Source: CAD feature listing. Evaluate the final solid. Frame: model axes, mm. A direction names the side the tool comes from. Give positions to 0.01 mm unless a question says otherwise; leave off trailing zeros. Order: outer loops, then holes, each group sorted by start corner. A loop starts at its lowest first (then second) coordinate and runs counter-clockwise, first axis right, second up. Notation, with made-up numbers: M 47.25,29.25 L 103.25,29.25 A10 ccw 103.25,37.25 Z; hole C -19.5,66.5 d6. An arc over 180 degrees is marked long. Answer as a JSON object with one key per item and string values. Group by question number.
1. Material intervals for L1, parallel to X at y = 78.5, z = -10; L2, parallel to X at y = 212.5, z = -2; L3, parallel to Z at x = 19.5, y = 117, sorted ascending. Write a range as [from, to].
2. Pin query (flat end, axial travel): P1, Ø0.8, axis at y = 140, z = -0.5, coming from the -X side; P2, Ø0.8, axis at y = 109.5, z = -0.5, coming from the +X side; P3, Ø1.5, axis at x = 29, y = 206.5, coming from the +Z side. Return the tip coordinate at first contact, or that it passes through.
3. Set-up query: faces 5 (the flat face through (6.2, 117, -10)), 6 (the flat face through (5.38, 116.84, -4.32)), 7 (the flat face through (4, 117, 0)). Return all of +Z, -Z, +X, -X, +Y, -Y with unobstructed straight access to the full face (end or side cutting, diameter ignored); none if empty.
4. Section query A-A (z = -10). Output: boundary loops of the cut face in (x, y), plus the area to 3 significant figures.
5. Section query C-C (y = 124). Count the separate pieces of the cut face and the enclosed holes in it, plus the area to 3 significant figures.
6. Section query B-B (x = 30). Output: boundary loops of the cut face in (y, z), plus the area to 3 significant figures.
7. Pull-direction query (Z, two-part tool) for faces 1 (the flat face through (35.68, 116.84, -5.38)), 2 (the flat face through (0, 117, -16)), 3 (the flat face through (24.34, 116.84, -5.38)), 4 (the flat face through (36, 117, -20)); classes: +Z half, -Z half, draft (parallel to the pull), parting line (faces both ways), or undercut.
from build123d import *

# Parameters (mm, degrees)
SKETCH1_R           = 2.1
BOSS_EXTRUDE1_DEPTH = 237
FILLET1_R           = 1.5


with BuildPart() as part:
    # Sketch1 → Boss-Extrude1 (new body)
    with BuildSketch(Plane(origin=(0, 0, 0), x_dir=(1, 0, 0), z_dir=(0, 1, 0))):
        Polygon((0, 0), (7, 0), (7, 1.5), (3.560660172, 1.5), (3.560660172, 2.5), (7.260660172, 6.2), (12.739339828, 6.2), (16.439339828, 2.5), (16.439339828, 1.5), (13, 1.5), (13, 0), (27, 0), (27, 1.5), (23.560660172, 1.5), (23.560660172, 2.5), (27.260660172, 6.2), (32.739339828, 6.2), (36.439339828, 2.5), (36.439339828, 1.5), (33, 1.5), (33, 0), (40, 0), (40, 7), (38.5, 7), (38.5, 3.560660172), (37.5, 3.560660172), (33.8, 7.260660172), (33.8, 12.739339828), (37.5, 16.439339828), (38.5, 16.439339828), (38.5, 13.45318801), (40, 13.45318801), (40, 20), (33, 20), (33, 18.5), (36.439339828, 18.5), (36.439339828, 17.5), (32.739339828, 13.8), (27.260660172, 13.8), (23.560660172, 17.5), (23.560660172, 18.5), (27, 18.5), (27, 20), (13, 20), (13, 18.5), (16.439339828, 18.5), (16.439339828, 17.5), (12.739339828, 13.8), (7.260660172, 13.8), (3.560660172, 17.5), (3.560660172, 18.5), (7, 18.5), (7, 20), (0, 20), (0, 13.45318801), (1.5, 13.45318801), (1.5, 16.439339828), (2.5, 16.439339828), (6.2, 12.739339828), (6.2, 7.260660172), (2.5, 3.560660172), (1.5, 3.560660172), (1.5, 7), (0, 7), align=None)
        with Locations(Location((10, 10, 0), (0, 0, 270))):
            Circle(SKETCH1_R, mode=Mode.SUBTRACT)
        with Locations(Location((30, 10, 0), (0, 0, 270))):
            Circle(SKETCH1_R, mode=Mode.SUBTRACT)
        Polygon((17.496963478, 16.458315541), (13.777987766, 12.739339828), (13.777987766, 7.260660172), (17.496963478, 3.541684459), (22.503036522, 3.541684459), (26.222012234, 7.260660172), (26.222012234, 12.739339828), (22.503036522, 16.458315541), align=None, mode=Mode.SUBTRACT)
    extrude(amount=BOSS_EXTRUDE1_DEPTH)

    # Fillet1
    fillet1_edges = [part.edges().sort_by_distance(p)[0] for p in [
        (40, 118.5, -20),
        (40, 118.5, 0),
        (0, 118.5, 0),
        (0, 118.5, -20),
    ]]
    fillet(fillet1_edges, radius=FILLET1_R)


solid = part.part
Answer sheet:
{
 "1": {"L1": "[6.2, 7.9], [12.1, 13.78], [26.22, 27.9], [32.1, 33.8]", "L2": "[0, 3.56], [16.44, 23.56], [36.44, 40]", "L3": "[-20, -16.46], [-3.54, 0]"},
 "2": {"P1": "x = 0.13", "P2": "x = 39.87", "P3": "z = -6.2"},
 "3": {"face 5": "-X, +Y, -Y", "face 6": "+Y, -Y", "face 7": "+Z, +X, -X, +Y, -Y"},
 "4": {"outline": "M 6.2,0 L 7.9,0 L 7.9,237 L 6.2,237 Z; M 12.1,0 L 13.78,0 L 13.78,237 L 12.1,237 Z; M 26.22,0 L 27.9,0 L 27.9,237 L 26.22,237 Z; M 32.1,0 L 33.8,0 L 33.8,237 L 32.1,237 Z", "area": "1,600 mm^2"},
 "5": {"separate pieces": "1", "enclosed holes": "3", "area": "301 mm^2"},
 "6": {"outline": "M 0,-13.8 L 237,-13.8 L 237,-12.1 L 0,-12.1 Z; M 0,-7.9 L 237,-7.9 L 237,-6.2 L 0,-6.2 Z", "area": "806 mm^2"},
 "7": {"face 1": "undercut", "face 2": "draft", "face 3": "undercut", "face 4": "-Z half"}
}
